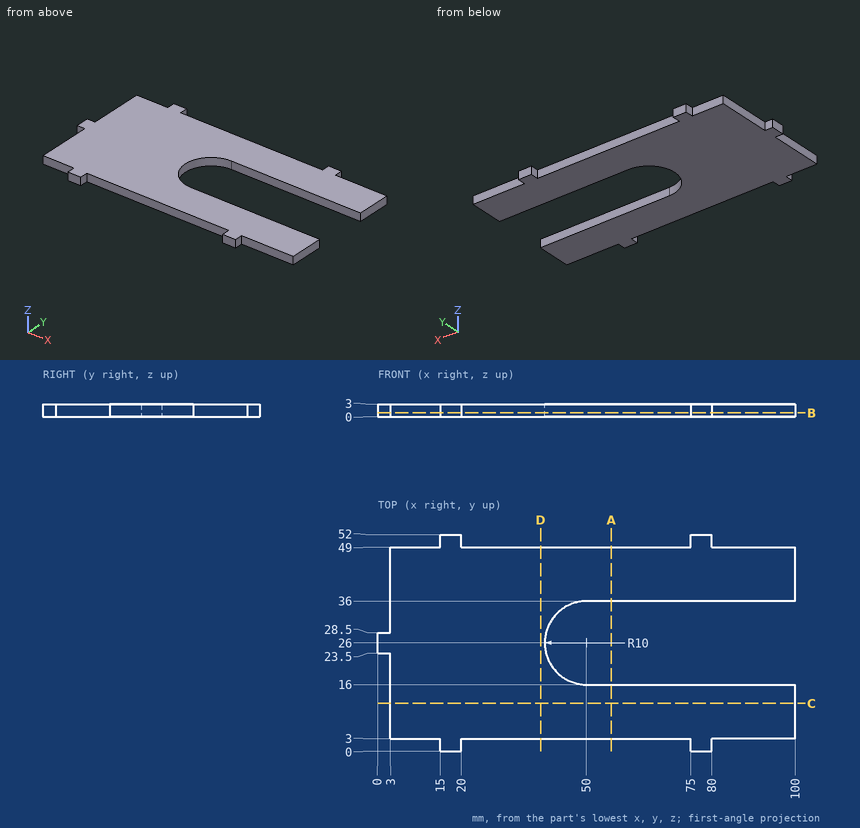
Job drawing, mm, ordinate dimensions from the low corner. One solid piece. Give positions to 0.01 mm unless a question says otherwise; leave off trailing zeros. Loops run counter-clockwise (first coordinate to the right, second up) from the corner with the lowest first, then second, coordinate; pieces in that order, holes last. Notation, with made-up numbers: M 56,-6 L 72,-6 A6 cw 72,3 Z; hole C -10,50 d4. An arc over 180 degrees is marked long. Put each result on its own line as item: value. Start each with the question number.
1) Saw through at B-B (z = 0.9). List the corners of the cut face in (x, y), then the cut area to 3 significant figures.
2) Saw through at D-D (x = 39). List the corners of the cut face in (y, z).
3) Saw through at C-C (y = 11.5). List the corners of the cut face in (x, z), then the cut area to 3 significant figures.
4) Saw through at A-A (x = 56). List the corners of the cut face in (y, z).
5) Probe probe 1 along Y at (x, z) = (79, 1.8); probe 2 along Y at (x, z) = (61, 0.65); probe 3 along X at (y, z) = (41, 2.5). List the from-to ranges inside material, lowest first.
6) Flat gauge pins, fed straight in: pin 1 (1.5 mm diameter, centred on x = 84.5, z = 1.5, fed in from +Y); pin 2 (1.5 mm diameter, centred on y = 2, z = 1.5, fed in from -X); pin 3 (0.9 mm diameter, centred on y = 50.5, z = 2, fed in from +X); pin 4 (12 mm diameter, centred on x = 33.5, y = 16.5, fed in from -Z). Where does each tip first touch, or does it go through?
Numbers:
1. outline: M 0,23.5 L 3,23.5 L 3,3 L 15,3 L 15,0 L 20,0 L 20,3 L 75,3 L 75,0 L 80,0 L 80,3 L 100,3 L 100,16 L 50,16 A10 cw 50,36 L 100,36 L 100,49 L 80,49 L 80,52 L 75,52 L 75,49 L 20,49 L 20,52 L 15,52 L 15,49 L 3,49 L 3,28.5 L 0,28.5 Z
1. area: 3,380 mm^2
2. outline: M 3,0 L 49,0 L 49,3 L 3,3 Z
3. outline: M 3,0 L 100,0 L 100,3 L 3,3 Z
3. area: 291 mm^2
4. outline: M 3,0 L 16,0 L 16,3 L 3,3 Z; M 36,0 L 49,0 L 49,3 L 36,3 Z
5. probe 1: 0 to 16, 36 to 52
5. probe 2: 3 to 16, 36 to 49
5. probe 3: 3 to 100
6. pin 1: y = 49
6. pin 2: x = 15
6. pin 3: x = 80
6. pin 4: z = 0
